Could you check a few things on this model? Use its own coordinates, in mm. Face numbers are marked on the shaded views. Give positions to 0.01 mm unless a question says otherwise; leave off trailing zeros. Loops run counter-clockwise (first coordinate to the right, second up) from the corner with the lowest first, then second, coordinate; pieces in that order, holes last. Notation, with made-up numbers: M 70,87 L 117,87 A29 cw 117,108 Z; hole C 26,-22 d2. An arc over 180 degrees is marked long. Return JSON: item names as keys, results as strings. Group by question number.
1. For pin 1 (2 mm diameter, centred on x = 15.5, y = 3.5, fed in from +Z); pin 2 (0.6 mm diameter, centred on x = 49.5, z = 3.5, fed in from +Y); pin 3 (1.8 mm diameter, centred on x = 45.5, y = 1, fed in from +Z), each with a flat end and sliding along its axis, tell me the tip position at first contact or that it passes through.
2. If we section it at A-A (y = 0): Write out the boundary of the cut face in (x, z).
3. If we mould it in two halves opening along X, with no side actions, what happens to the marked faces 1, 2 and 3? For each: +X half, -X half, draft (parallel to the pull), parting line (faces both ways), or undercut.
4. Please list where these lines run through material, in increasing order: line 1 (Z direction, x = 15, y = -4); line 2 (Y direction, x = 41.5, z = 0); line 3 (Z direction, x = 43.5, y = 0).
5. If we section it at B-B (z = 0): Write out the boundary of the cut face in (x, y).
6. If we section it at C-C (x = 30.5): Write out the boundary of the cut face in (y, z), plus the area to 3 significant figures.
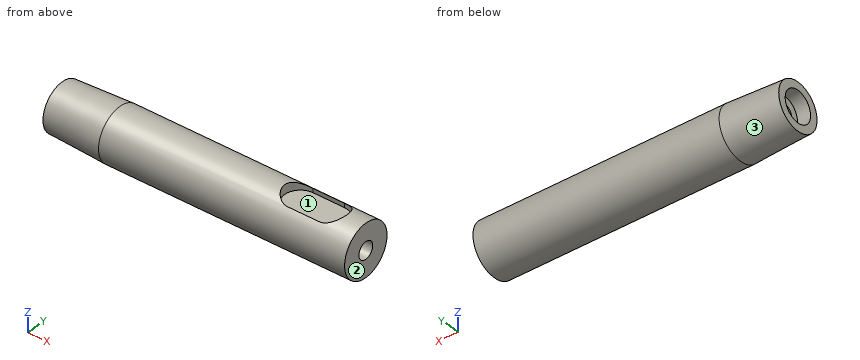
Autodesk Inventor part; units mm, degrees
ref_plane "Arbeitsebene1" through (0, 0, 5) normal (0, 0, 1) x (1, 0, 0)
ref_plane "YZ Plane" through (0, 0, 0) normal (1, 0, 0) x (0, 1, 0)
ref_plane "XZ Plane" through (0, 0, 0) normal (0, 1, 0) x (-1, 0, 0)
sketch "Skizze1" plane through (0, 0, 0) normal (0, 0, 1) x (1, 0, 0)
  line L0 (0, 0) -> (0, 4.5197)
  line L1 (0, 4.5197) -> (11, 5)
  line L2 (11, 5) -> (58, 5)
  line L3 (58, 5) -> (58, 0)
  line L4 (58, 0) -> (0, 0)
  dimension "d0" = 2.5
  dimension "d1" = 58
  dimension "d2" = 10
  dimension "d3" = 11
revolve "Umdrehung1" add sketch "Skizze1" angle 360 about axis through (58, 0, 0) along (-1, 0, 0)
ref_plane "Arbeitsebene1" through (0, 0, 5) normal (0, 0, 1) x (1, 0, 0)
sketch "Skizze2" plane through (0, 0, 5) normal (0, 0, 1) x (1, 0, 0)
  line L0 (58, 5) -> (58, -5)
  line L1 (0, 0) -> (78.1266, 0) construction
  line L2 (45.5, 0) -> (51.5, 0) construction
  line L3 (45.5, -3) -> (51.5, -3)
  line L4 (51.5, 3) -> (45.5, 3)
  arc A0 (45.5, 3) -> (45.5, -3) centre (45.5, 0) ccw
  arc A1 (51.5, -3) -> (51.5, 3) centre (51.5, 0) ccw
  point P0 (48.5, 0)
  point P1 (58, 0)
  point P2 (54.5, 0)
  point P3 (42.5, 0)
  dimension "d8" = 12
  dimension "d9" = 3.5
  dimension "d10" = 3
extrude "Extrusion1" cut sketch "Skizze2" against normal blind 1.8
sketch "Skizze3" plane through (0, 0, 0) normal (-1, 0, 0) x (0, 0, 1)
  circle A0 centre (0, 0) radius 4.5197
hole "Bohrung1" at (0, 0, 0) direction (1, 0, 0) diameter 3.242 depth 58 counterbore diameter 6 counterbore depth 2.5
properties part number "Welle" material "Aluminum 6061-AHC"
Answer:
{
 "1": {"pin 1": "stops at z = 4.33", "pin 2": "stops at y = 3.84", "pin 3": "stops at z = 3.2"},
 "2": {"outline": "M 0,-4.52 L 11,-5 L 58,-5 L 58,-1.62 L 2.5,-1.62 L 2.5,-3 L 0,-3 Z; M 0,3 L 2.5,3 L 2.5,1.62 L 58,1.62 L 58,5 L 54.5,5 L 54.5,3.2 L 42.5,3.2 L 42.5,5 L 11,5 L 0,4.52 Z"},
 "3": {"face 1": "undercut", "face 2": "+X half", "face 3": "-X half"},
 "4": {"line 1": "z = -3 to 3", "line 2": "y = -5 to -1.62, 1.62 to 5", "line 3": "z = -5 to -1.62, 1.62 to 3.2"},
 "5": {"outline": "M 0,-4.52 L 11,-5 L 58,-5 L 58,-1.62 L 2.5,-1.62 L 2.5,-3 L 0,-3 Z; M 0,3 L 2.5,3 L 2.5,1.62 L 58,1.62 L 58,5 L 11,5 L 0,4.52 Z"},
 "6": {"outline": "C 0,0 d10; hole C 0,0 d3.24", "area": "70.3 mm²"}
}
